Source: CAD feature listing. Evaluate the final solid. Frame: model axes, mm. A direction names the side the tool comes from. Round coordinates to 2 decimals unless told otherwise and drop trailing zeros. Loops run counter-clockwise (first coordinate to the right, second up) from the corner with the lowest first, then second, coordinate; pieces in that order, holes last. Notation, with made-up numbers: (26, 8) - (71, 8) arc R24 cw to (71, 24) - close; hole circle Ø3 at (-28.75, -12.5). An arc over 180 degrees is marked (long way). One line per question, with ' | ' between items. Start each with the question number.
1. Pin query (flat end, axial travel): pin 1 (2 mm diameter, centred on x = -12.5, y = 3.5, fed in from +Z); pin 2 (10 mm diameter, centred on x = 23.5, z = 1, fed in from +Y); pin 3 (1.5 mm diameter, centred on y = 5, z = 17, fed in from +X); pin 4 (5.5 mm diameter, centred on x = 0, z = -17.5, fed in from -Y). Return the tip coordinate at first contact, or that it passes through.
2. Cut plane B-B (y = 4.7). Return loops of the section in (x, z), then the cut area to 3 significant figures.
3. Mould query, pull axis Z, two halves, no side actions, for faces 4 (the cylindrical face through (28, 3, -9)), 5 (the cylindrical face through (24.5, 3, 0.1)), 6 (the flat face through (-7, 3, 17)). Classes: pulls with the +Z half, pulls with the -Z half, needs draft (parallel to the pull), parting line crosses it, or undercut.
4. Cut plane C-C (x = 22). Return loops of the section in (y, z).
5. Access query for faces 1 (the flat face through (-7, 3, -17)), 2 (the flat face through (7, 3, 17)), 3 (the flat face through (-18, 3, 10)). Directions: +Z, -Z, +X, -X, +Y, -Y. A direction counts if a zero-diameter tool reaches every point of the face in a straight line with its end or side. Return the directions, or none.
6. Ray query, line 1 (Z direction, x = 0, y = 3.9); line 2 (Z direction, x = 22, y = 2.25); line 3 (Z direction, x = 16.5, y = 5.2). Return the intervals inside material, ascending.
7. Cut plane D-D (z = 17.5). Return loops of the section in (x, y), then the cut area to 3 significant figures.
8. Cut plane A-A (z = 0). Return loops of the section in (x, y), then the cut area to 3 significant figures.
```python
from build123d import *

# Parameters (mm, degrees)
F1_DEPTH = 6
F2_D     = 6
F3_D     = 5
F4_R     = 5


with BuildPart() as f1:
    # F0 (on Front) → F1 (new body)
    with BuildSketch(Plane.XZ):
        Polygon((-7, -24.5), (7, -24.5), (7, -10), (30, -10), (30, 10), (7, 10), (7, 24.5), (-7, 24.5), (-7, 10), (-30, 10), (-30, -10), (-7, -10), align=None)
    extrude(amount=-F1_DEPTH)

    # F2 (through all)
    with Locations(Plane.XZ):
        with Locations((0, 17.5), (0, -17.5)):
            Hole(F2_D / 2)

    # F3 (through all)
    with Locations(Plane.XZ):
        with Locations((22, 0), (-22, 0)):
            Hole(F3_D / 2)

    # F4
    f4_edges = [f1.edges().sort_by_distance(p)[0] for p in [
        (7, 3, 24.5),
        (7, 3, 10),
        (30, 3, 10),
        (30, 3, -10),
        (7, 3, -24.5),
        (7, 3, -10),
        (-7, 3, -24.5),
        (-30, 3, -10),
        (-7, 3, -10),
        (-30, 3, 10),
        (-7, 3, 10),
        (-7, 3, 24.5),
    ]]
    fillet(f4_edges, radius=F4_R)


solid = f1.part
```
Answers follow:
1) pin 1: stops at z = 10.03 | pin 2: stops at y = 6 | pin 3: stops at x = 7 | pin 4: passes through
2) outline: (-30, -5) arc R5 ccw to (-25, -10) - (-12, -10) arc R5 cw to (-7, -15) - (-7, -19.5) arc R5 ccw to (-2, -24.5) - (2, -24.5) arc R5 ccw to (7, -19.5) - (7, -15) arc R5 cw to (12, -10) - (25, -10) arc R5 ccw to (30, -5) - (30, 5) arc R5 ccw to (25, 10) - (12, 10) arc R5 cw to (7, 15) - (7, 19.5) arc R5 ccw to (2, 24.5) - (-2, 24.5) arc R5 ccw to (-7, 19.5) - (-7, 15) arc R5 cw to (-12, 10) - (-25, 10) arc R5 ccw to (-30, 5) - close; hole circle Ø5 at (-22, 0); hole circle Ø6 at (0, -17.5); hole circle Ø6 at (0, 17.5); hole circle Ø5 at (22, 0) | area: 1,490 mm2
3) face 4: pulls with the -Z half | face 5: undercut | face 6: needs draft
4) outline: (0, -10) - (6, -10) - (6, -2.5) - (0, -2.5) - close; (0, 2.5) - (6, 2.5) - (6, 10) - (0, 10) - close
5) face 1: -Z, -X, +Y, -Y | face 2: +Z, +X, +Y, -Y | face 3: +Z, -X, +Y, -Y
6) line 1: z = -24.5 to -20.5, -14.5 to 14.5, 20.5 to 24.5 | line 2: z = -10 to -2.5, 2.5 to 10 | line 3: z = -10 to 10
7) outline: (-7, 0) - (-3, 0) - (-3, 6) - (-7, 6) - close; (3, 0) - (7, 0) - (7, 6) - (3, 6) - close | area: 48.0 mm2
8) outline: (-30, 0) - (-24.5, 0) - (-24.5, 6) - (-30, 6) - close; (-19.5, 0) - (19.5, 0) - (19.5, 6) - (-19.5, 6) - close; (24.5, 0) - (30, 0) - (30, 6) - (24.5, 6) - close | area: 300 mm2
